Answer from the drawing. Dimensions are ordinates in mm from the lowest x, y and z of the part. Give positions to 0.01 mm unless a question says otherwise; leave off trailing zeros. Order: outer loops, then holes, each group sorted by start corner. A loop starts at its lowest first (then second) coordinate and runs counter-clockwise, first axis right, second up. Notation, with made-up numbers: (89.25, 8.25) -> (98.25, 8.25) arc R20 cw to (98.25, 27.25) -> close; hole circle Ø3 at (62.5, 58.25). An arc over 180 degrees is marked (long way). Answer as CSV lines item,"result". Start each with the question number.
1) Find section A-A (y = 10). Determine the outline of the cut face in (x, z).
2) Find section C-C (z = 4.2). Determine the outline of the cut face in (x, y).
3) Find section B-B (x = 76.5). Determine the outline of the cut face in (y, z), and give its area (4 significant figures).
4) Find section D-D (y = 59). Determine the outline of the cut face in (x, z), and give its area (4 significant figures).
5) Straight lines are drawn through the part: L1, parallel to X at y = 59, z = 1.1; L2, parallel to Y at x = 12, z = 0.9; L3, parallel to X at y = 34, z = 1.35. For each, find the intervals that lie inside material, in ascending order. Write a range as from..to.
6) Flat-ended cylindrical pins translate along their axes: pin 1 Ø5.5 at (x, y) = (37, 59) entering from +Z; pin 2 Ø0.9 at (y, z) = (42.5, 3.5) entering from -X; pin 3 Ø2.5 at (y, z) = (59, 1.5) entering from -X; pin 4 Ø0.9 at (x, z) = (29, 1.5) entering from +Y. Find the tip coordinate at first contact, or state that the pin passes through.
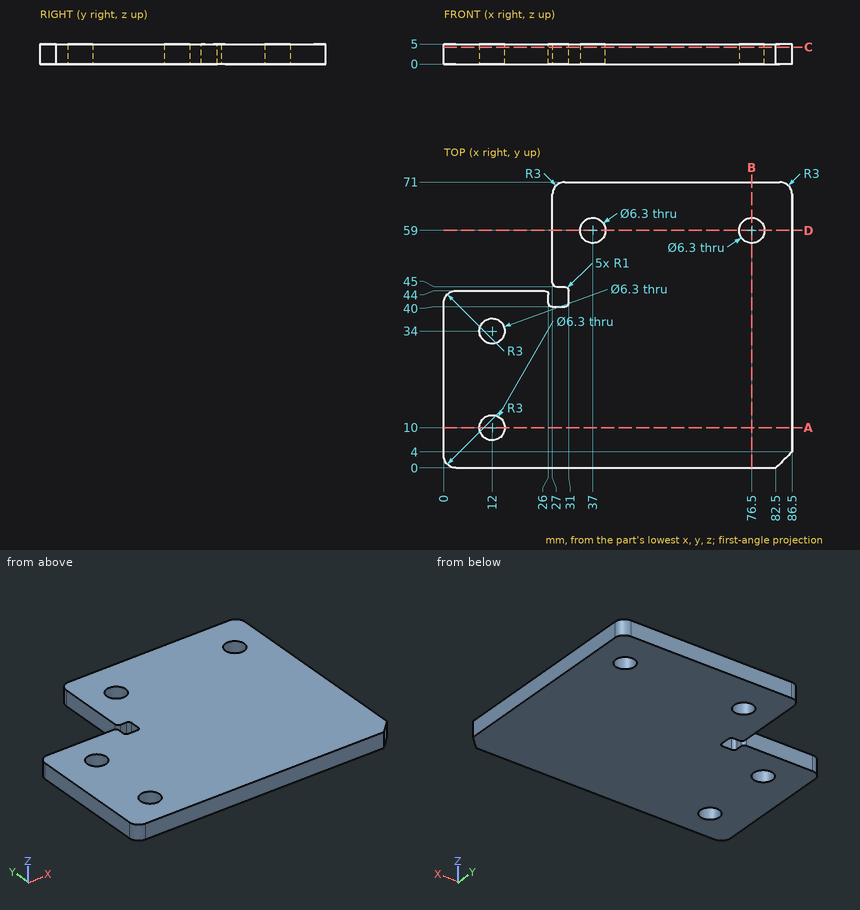
Findings below:
1,outline,"(0, 0) -> (8.85, 0) -> (8.85, 5) -> (0, 5) -> close; (15.15, 0) -> (86.5, 0) -> (86.5, 5) -> (15.15, 5) -> close"
2,outline,"(0, 3) arc R3 ccw to (3, 0) -> (82.5, 0) -> (86.5, 4) -> (86.5, 68) arc R3 ccw to (83.5, 71) -> (30, 71) arc R3 ccw to (27, 68) -> (27, 46) arc R1 ccw to (28, 45) -> (30, 45) arc R1 cw to (31, 44) -> (31, 41) arc R1 cw to (30, 40) -> (27, 40) arc R1 cw to (26, 41) -> (26, 43) arc R1 ccw to (25, 44) -> (3, 44) arc R3 ccw to (0, 41) -> close; hole circle Ø6.3 at (12, 10); hole circle Ø6.3 at (12, 34); hole circle Ø6.3 at (37, 59); hole circle Ø6.3 at (76.5, 59)"
3,outline,"(0, 0) -> (55.85, 0) -> (55.85, 5) -> (0, 5) -> close; (62.15, 0) -> (71, 0) -> (71, 5) -> (62.15, 5) -> close"
3,area,"323.5 mm²"
4,outline,"(27, 0) -> (33.85, 0) -> (33.85, 5) -> (27, 5) -> close; (40.15, 0) -> (73.35, 0) -> (73.35, 5) -> (40.15, 5) -> close; (79.65, 0) -> (86.5, 0) -> (86.5, 5) -> (79.65, 5) -> close"
4,area,"234.5 mm²"
5,L1,"27..33.85, 40.15..73.35, 79.65..86.5"
5,L2,"0..6.85, 13.15..30.85, 37.15..44"
5,L3,"0..8.85, 15.15..86.5"
6,pin 1,"through"
6,pin 2,"x = 0.19"
6,pin 3,"x = 27"
6,pin 4,"y = 70.95"
